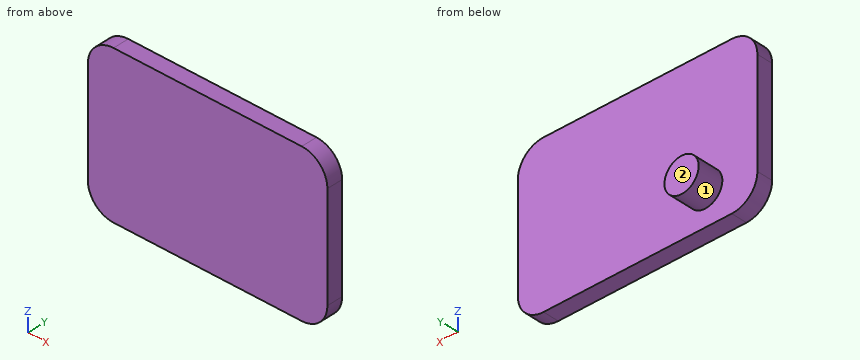
```python
from build123d import *

# Parameters (mm, degrees)
SKETCH1_W           = 1422.4
SKETCH1_H           = 924.56
BOSS_EXTRUDE1_DEPTH = 94.826666667
FILLET1_R           = 152.4
SKETCH1_3_R         = 101.6
BOSS_EXTRUDE2_DEPTH = 152.4


with BuildPart() as part:
    # Sketch1 → Boss-Extrude1 (new body)
    with BuildSketch(Plane(origin=(0, 0, 0), x_dir=(1, 0, 0), z_dir=(0, 1, 0))):
        Rectangle(SKETCH1_W, SKETCH1_H)
    extrude(amount=-BOSS_EXTRUDE1_DEPTH)

    # Fillet1
    fillet1_edges = [part.edges().sort_by_distance(p)[0] for p in [
        (-711.2, -47.413333333, 462.28),
        (711.2, -47.413333333, 462.28),
        (711.2, -47.413333333, -462.28),
        (-711.2, -47.413333333, -462.28),
    ]]
    fillet(fillet1_edges, radius=FILLET1_R)

    # Sketch1_3 → Boss-Extrude2 (add)
    with BuildSketch(Plane(origin=(0, 0, 0), x_dir=(1, 0, 0), z_dir=(0, 1, 0))):
        with Locations(Location((-401.553909641, 261.010041267, 0), (0, 0, 90))):
            Circle(SKETCH1_3_R)
    extrude(amount=BOSS_EXTRUDE2_DEPTH)


solid = part.part
```
Can you work these out from the model? Positions are in its coordinate system, mm. Face numbers are marked on the shaded views. A direction names the side the tool comes from. Give positions to 0.01 mm unless a question says otherwise; leave off trailing zeros. Loops run counter-clockwise (first coordinate to the right, second up) from the corner with the lowest first, then second, coordinate; pieces in that order, holes last. Notation, with made-up numbers: M -10,-15 L -4,-15 A22 cw -4,18 Z; hole C 18.25,42 d10. An arc over 180 degrees is marked long. Answer in a Markdown table with one row per item.
1. Which directions (+Z, -Z, +X, -X, +Y, -Y) give clear straight access to the entire face, cutting with the end or side of a thin tool? Please do the marked faces 1 and 2.
Taken from the geometry:
| item | result |
|---|---|
| face 1 | +Y |
| face 2 | +Z, -Z, +X, -X, +Y |
2. Suppose I cut it at A-A on z = -242.5. Write out the boundary of the cut face in (x, y), plus the area to 3 significant figures.
Taken from the geometry:
| item | result |
|---|---|
| outline | M -711.2,-94.83 L 711.2,-94.83 L 711.2,0 L -301.65,0 L -301.65,152.4 L -501.45,152.4 L -501.45,0 L -711.2,0 Z |
| area | 165,000 mm² |
3. If I drill on line 1 along Y through (x, z) = (208.5, 105); line 2 along X through (y, z) = (37, -180); line 3 along X through (y, z) = (62.5, -185), over which ranges is the centre line in solid material (lowest first)?
Taken from the geometry:
| item | result |
|---|---|
| line 1 | y = -94.83 to 0 |
| line 2 | x = -462.87 to -340.24 |
| line 3 | x = -468.97 to -334.14 |
4. Suppose I cut it at C-C on y = 69. Write out the boundary of the cut face in (x, z).
Taken from the geometry:
| item | result |
|---|---|
| outline | C -401.55,-261.01 d203.2 |
5. Suppose I cut it at D-D on z = 239. Write out the boundary of the cut face in (x, y), plus the area to 3 significant figures.
Taken from the geometry:
| item | result |
|---|---|
| outline | M -711.2,-94.83 L 711.2,-94.83 L 711.2,0 L -711.2,0 Z |
| area | 135,000 mm² |
6. Suppose I cut it at B-B on x = 423.5. Write out the boundary of the cut face in (y, z), plus the area to 3 significant figures.
Taken from the geometry:
| item | result |
|---|---|
| outline | M -94.83,-462.28 L 0,-462.28 L 0,462.28 L -94.83,462.28 Z |
| area | 87,700 mm² |
7. For pin 1 Ø2 at (x, z) = (-151.5, -331.5) entering from +Y, with a flat end and sliding along its axis, tell me the tip position at first contact or that it passes through.
Taken from the geometry:
| item | result |
|---|---|
| pin 1 | stops at y = 0 |
